Read the model definition and answer for the solid it produces. Units are mm, in the model's axes. A direction names the side the tool comes from. Give positions to 0.01 mm unless a question says otherwise; leave off trailing zeros. Loops run counter-clockwise (first coordinate to the right, second up) from the corner with the lowest first, then second, coordinate; pieces in that order, holes last. Notation, with made-up numbers: (51.25, 85.5) - (80.25, 85.5) arc R20 cw to (80.25, 112.5) - close; hole circle Ø7 at (73.25, -6). An arc over 180 degrees is marked (long way). Use a Markdown table: item, result. Add a question column.
Item 1: A cutting plane is placed at D-D (y = 2.5). Determine the outline of the cut face in (x, z), plus the area to 3 significant figures.
Item 2: A cutting plane is placed at A-A (y = -1). Determine the outline of the cut face in (x, z).
Item 3: Which of the six approach directions +Z, -Z, +X, -X, +Y, -Y give full straight-line access (tool end or side, diameter ignored) to faces 4 (the face through (-2.5, 10.2, 9.7)), 5 (the face through (3.7, 5.9, 11.1)), 6 (the face through (2, 0, 0)), 7 (the face through (-1.2, 2.75, 5.03)), 8 (the face through (-0.35, 7, 11))?
Item 4: A cutting plane is placed at C-C (z = 18.5). Determine the outline of the cut face in (x, y).
Item 5: Each of these flat-tipped pins is pushed along its axis until it touches: P1, Ø8, axis at y = 9, z = 11, coming from the -X side; P2, Ø1, axis at y = -1.5, z = 10.5, coming from the +X side; P3, Ø6, axis at y = 9.5, z = 12, coming from the -X side; P4, Ø1.9, axis at x = 0, y = 0, coming from the -Z side. Where does it stop, or does it pass through?
Item 6: A cutting plane is placed at B-B (z = 11). Determine the outline of the cut face in (x, y).
Item 7: For a pull along Y with two mould halves and no side action, classify faces 1 (the face through (2.14, 9.96, 17.62)), 2 (the face through (-3, 11.685, 11)), 3 (the face through (1.386, -4.695, 4.425)) as +Y half, -Y half, draft (parallel to the pull), parting line (faces both ways), or undercut.
Item 8: Consider probe 1 along X at (y, z) = (0, 1.35); probe 2 along Y at (x, z) = (0.9, 11); probe 3 along Y at (x, z) = (0, 16.25). Determine where each line is inside the solid, lowest interval first. Write a range as [from, to].
from build123d import *

# Parameters (mm, degrees)
EXTRUDE003_DEPTH                     = 10
SKETCH005_R                          = 3.1
EXTRUDE002_DEPTH                     = 10
SKETCH003_AS_DRAWN_R                 = 1.5
EXTRUDE001_DEPTH                     = 10
EXTRUDE001_ONTO_SKETCH003_ROLL_ANGLE = 90
EXTRUDE_DEPTH                        = 22
SKETCH001_R                          = 5
POCKET_DEPTH                         = 15
SKETCH002_R                          = 3
POCKET001_DEPTH                      = 4
FILLET_R                             = 0.35
SKETCH004_R                          = 1.55
POCKET002_DEPTH                      = 6.651
POCKET002_DEPTH_BACK                 = -7.351
FILLET001_R                          = 2


with BuildPart() as extrude003:
    # Sketch006 → Extrude003 (new body)
    with BuildSketch(Plane(origin=(-2.5, 0, 0), x_dir=(0, -1, 0), z_dir=(-1, 0, 0))):
        Polygon((-9, 14.1), (-11.684679, 12.55), (-11.684679, 9.45), (-9, 7.9), (-6.315321, 9.45), (-6.315321, 12.55), align=None)
    extrude(amount=EXTRUDE003_DEPTH)


with BuildPart() as extrude002:
    # Sketch005 → Extrude002 (new body)
    with BuildSketch(Plane.YZ.offset(2.5)):
        with Locations((9, 11)):
            Circle(SKETCH005_R)
    extrude(amount=EXTRUDE002_DEPTH)


with BuildPart() as extrude001:
    # Sketch003 as drawn → Extrude001 (new)
    with BuildSketch(Plane.XY):
        with Locations((0, 5)):
            Circle(SKETCH003_AS_DRAWN_R)
    extrude(amount=EXTRUDE001_DEPTH)


with BuildPart() as extrude001_1:
    # Extrude001 onto Sketch003 roll: moved
    add(extrude001.part.rotate(Axis((0, 0, 0), (1, 0, 0)), EXTRUDE001_ONTO_SKETCH003_ROLL_ANGLE))


with BuildPart() as extrude001_2:
    # Extrude001 onto Sketch003 placement: moved
    add(extrude001_1.part)


with BuildPart() as fillet001:
    # Sketch → Extrude (new body)
    with BuildSketch(Plane.XY):
        with BuildLine():
            ThreePointArc((-0.35, 1.509967), (0, -1.55), (0.35, 1.509967))
            Line((0.35, 1.509967), (0.35, 13))
            Line((0.35, 13), (3.35, 13))
            Line((3.35, 13), (6.694934, 2.043982))
            ThreePointArc((-6.694921, 2.044024), (-2.2e-05, -7), (6.694934, 2.043982))
            Line((-6.694921, 2.044024), (-3.35, 13))
            Line((-3.35, 13), (-0.35, 13))
            Line((-0.35, 13), (-0.35, 1.509967))
        make_face()
    extrude(amount=EXTRUDE_DEPTH)

    # Sketch001 → Pocket (cut)
    with BuildSketch(Plane.XY.offset(22)):
        Circle(SKETCH001_R)
    extrude(amount=-POCKET_DEPTH, mode=Mode.SUBTRACT)

    # Sketch002 → Pocket001 (cut)
    with BuildSketch(Plane.XY.offset(7)):
        Circle(SKETCH002_R)
    extrude(amount=-POCKET001_DEPTH, mode=Mode.SUBTRACT)

    # Cut: cut Extrude001
    add(extrude001_2.part, mode=Mode.SUBTRACT)

    # Fillet
    fillet_edges = [fillet001.edges().sort_by_distance(p)[0] for p in [
        (-1.5, -6.837397, 5),
        (-1.5, -2.598076, 5),
    ]]
    fillet(fillet_edges, radius=FILLET_R)

    # Sketch004 → Pocket002 (cut, two sides)
    with BuildSketch(Plane.YZ.offset(-0.35)) as pocket002_sk:
        with Locations((8.993867, 11)):
            Circle(SKETCH004_R)
        Polygon((6.987735, 22), (6.987735, 21.165138), (13, 14), (13, 22), align=None)
        Polygon((13, 8), (6.987735, 0.834862), (6.987735, 0), (13, 0), align=None)
    extrude(amount=-POCKET002_DEPTH, mode=Mode.SUBTRACT)
    extrude(pocket002_sk.sketch, amount=-POCKET002_DEPTH_BACK, mode=Mode.SUBTRACT)

    # Cut001: cut Extrude002
    add(extrude002.part, mode=Mode.SUBTRACT)

    # Cut003: cut Extrude003
    add(extrude003.part, mode=Mode.SUBTRACT)

    # Fillet001
    fillet001_edges = [fillet001.edges().sort_by_distance(p)[0] for p in [
        (-2.767789, 6.987735, 0.834862),
        (-1.85, 13, 8),
        (-2.767789, 6.987735, 21.165138),
        (-1.85, 13, 14),
        (2.767789, 6.987735, 0.834862),
        (2.767789, 6.987735, 21.165138),
        (1.85, 13, 8),
        (1.85, 13, 14),
    ]]
    fillet(fillet001_edges, radius=FILLET001_R)


solid = fillet001.part
Geometry says:
| question | item | result |
|---|---|---|
| 1 | outline | (-6.56, 0) - (-0.35, 0) - (-0.35, 3) - (-1.66, 3) - (-1.66, 7) - (-4.33, 7) - (-4.33, 22) - (-6.56, 22) - close; (0.35, 0) - (6.56, 0) - (6.56, 22) - (4.33, 22) - (4.33, 7) - (1.66, 7) - (1.66, 3) - (0.35, 3) - close |
| 1 | area | 143 mm² |
| 2 | outline | (-6.93, 0) - (-1.18, 0) - (-1.18, 3) - (-2.83, 3) - (-2.83, 7) - (-4.9, 7) - (-4.9, 22) - (-6.93, 22) - close; (1.18, 0) - (6.93, 0) - (6.93, 22) - (4.9, 22) - (4.9, 7) - (2.83, 7) - (2.83, 3) - (1.18, 3) - close |
| 3 | face 4 | -X |
| 3 | face 5 | +X |
| 3 | face 6 | -Z, +X, -X, +Y, -Y |
| 3 | face 7 | +Z |
| 3 | face 8 | +Z, -Z, +Y |
| 4 | outline | (-6.69, 2.04) arc R7 ccw (long way) to (6.69, 2.04) - (4.5, 9.22) - (0.35, 9.22) - (0.35, 4.99) arc R5 cw (long way) to (-0.35, 4.99) - (-0.35, 9.22) - (-4.5, 9.22) - close |
| 5 | P1 | x = -5.79 |
| 5 | P2 | x = 6.93 |
| 5 | P3 | x = -5.31 |
| 5 | P4 | through |
| 6 | outline | (-6.69, 2.04) arc R7 ccw (long way) to (6.69, 2.04) - (5.52, 5.9) - (2.5, 5.9) - (2.5, 7.44) - (0.35, 7.44) - (0.35, 4.99) arc R5 cw (long way) to (-0.35, 4.99) - (-0.35, 7.44) - (-2.5, 7.44) - (-2.5, 6.32) - (-5.39, 6.32) - close; (-3.75, 11.68) - (-2.5, 11.68) - (-2.5, 10.54) - (-0.35, 10.54) - (-0.35, 13) - (-3.35, 13) - close; (0.35, 10.54) - (2.5, 10.54) - (2.5, 12.1) - (3.62, 12.1) - (3.35, 13) - (0.35, 13) - close |
| 7 | face 1 | +Y half |
| 7 | face 2 | undercut |
| 7 | face 3 | draft |
| 8 | probe 1 | [-7, -1.55], [1.55, 7] |
| 8 | probe 2 | [-6.94, -4.92], [4.92, 7.44], [10.54, 13] |
| 8 | probe 3 | [-7, -5] |
